Geometry: final body of the model. Coordinates: model frame, mm. Give positions to 0.01 mm unless a question says otherwise; leave off trailing zeros. Loops run counter-clockwise (first coordinate to the right, second up) from the corner with the lowest first, then second, coordinate; pieces in that order, holes last. Notation, with made-up numbers: (87, -10) -> (95, -10) arc R18 ccw to (95, -5) -> close; hole circle Ø4 at (68, 60.25). An arc over 180 degrees is marked (long way). One line per question, with ' | ' between items. Start each with the question number.
Item 1: Pin query (flat end, axial travel): P1, Ø4, axis at x = -24.5, y = 1.5, coming from the -Z side; P2, Ø3, axis at x = -38, y = 0, coming from the -Z side; P3, Ø1.5, axis at x = 7, y = 4, coming from the +Z side. Return the tip coordinate at first contact, or that it passes through.
Item 2: Material intervals for line 1 along Y through (x, z) = (-38, 20); line 2 along X through (y, z) = (1, 18.75); line 3 along X through (y, z) = (-2.5, 19.25), sorted ascending. Write a range as [from, to].
Item 3: Section A-A on z = 18. Return loops of the section in (x, y).
from build123d import *

# Parameters (mm, degrees)
SALIENTE_EXTRUIR2_DEPTH      = 5
CROQUIS6_R                   = 3
SALIENTE_EXTRUIR3_DEPTH      = 10
CROQUIS7_R                   = 1.75
CORTAR_EXTRUIR1_DEPTH        = 10
CHAFL_N1_SIZE                = 2
REDONDEO2_START              = -5.0000001
REDONDEO2_DEPTH              = 10.0000002
SALIENTE_EXTRUIR8_DEPTH      = 4.62
SALIENTE_EXTRUIR8_DEPTH_BACK = 4.62
CROQUIS17_R                  = 2.5


with BuildPart() as part:
    # Croquis5 → Saliente-Extruir2 (new, symmetric)
    with BuildSketch(Plane(origin=(0, 0, 0), x_dir=(1, 0, 0), z_dir=(0, 1, 0))):
        with BuildLine():
            Line((0, -26), (0, -30))
            add(Edge.make_bspline(
                [(0, -30), (3.306526268, -30), (16.53263134, -29.831217065), (35.997648536, -28.565345051), (52.057120801, -26.333176426), (58.766277483, -25.109762555), (60, -24.873829164)],
                knots=[4.71238898, 4.71238898, 4.71238898, 4.71238898, 4.810563751, 5.105088062, 5.301437603, 5.346535107, 5.346535107, 5.346535107, 5.346535107], degree=3))
            Line((60, -24.873829164), (60, -20.8))
            add(Edge.make_bspline(
                [(0, -26), (33.333333333, -26), (60, -20.8)],
                knots=[4.71238898, 4.71238898, 4.71238898, 5.355890089, 5.355890089, 5.355890089], degree=2, weights=[1, 0.948683298, 1]))
        make_face()
    extrude(amount=SALIENTE_EXTRUIR2_DEPTH, both=True)

    # Croquis6 → Saliente-Extruir3 (add)
    with BuildSketch(Plane.XY.offset(26)):
        with Locations((38, 0)):
            Circle(CROQUIS6_R)
    extrude(amount=-SALIENTE_EXTRUIR3_DEPTH)

    # Croquis7 → Cortar-Extruir1 (cut)
    with BuildSketch(Plane(origin=(0, 0, 16), x_dir=(-1, 0, 0), z_dir=(0, 0, -1))):
        with Locations((-38, 0)):
            Circle(CROQUIS7_R)
    extrude(amount=-CORTAR_EXTRUIR1_DEPTH, mode=Mode.SUBTRACT)

    # Chaflán1
    chafl_n1_edges = [part.edges().sort_by_distance(p)[0] for p in [
        (60, -5, 22.836914582),
        (60, 5, 22.836914582),
        (30.12007931, -5, 28.805559056),
        (30.12007931, 5, 28.805559056),
    ]]
    chamfer(chafl_n1_edges, length=CHAFL_N1_SIZE)

    # Redondeo2: read off the stored shape, not the designer's step
    # Redondeo2 outline → Redondeo2 (cut)
    with BuildSketch(Plane(origin=(0, 0, 0), x_dir=(1, 0, 0), z_dir=(0, 1, 0)).offset(REDONDEO2_START)):
        with BuildLine():
            Line((60, -24.873829164), (60, -22.378802425))
            ThreePointArc((60, -22.378802425), (59.301153244, -24.303560526), (57.530204169, -25.331577991))
            add(Edge.make_bspline(
                [(57.530204169, -25.331577991), (58.36173126, -25.182267919), (59.185100773, -25.029668046), (60, -24.873829164)],
                knots=[5.316747273, 5.316747273, 5.316747273, 5.316747273, 5.346535107, 5.346535107, 5.346535107, 5.346535107], degree=3))
        make_face()
    extrude(amount=REDONDEO2_DEPTH, mode=Mode.SUBTRACT)

    # Croquis17 → Saliente-Extruir8 (add, two sides: drawn at the far end of the back side and taken through both)
    with BuildSketch(Plane(origin=(0, 0, 0), x_dir=(0, 0, -1), z_dir=(1, 0, 0)).offset(-SALIENTE_EXTRUIR8_DEPTH_BACK)):
        with BuildLine():
            ThreePointArc((-21.96097599, 5), (-16.96097599, 0), (-21.96097599, -5))
            Line((-21.96097599, -5), (-26.96097599, -5))
            Line((-26.96097599, -5), (-26.96097599, 5))
            Line((-26.96097599, 5), (-21.96097599, 5))
        make_face()
        with Locations((-21.96097599, 0)):
            Circle(CROQUIS17_R, mode=Mode.SUBTRACT)
    extrude(amount=SALIENTE_EXTRUIR8_DEPTH + SALIENTE_EXTRUIR8_DEPTH_BACK)

    # Simetría2: part across plane


with BuildPart() as part_1:
    add(part.part)
    add(part.part.mirror(Plane(origin=(0, 0, 0), x_dir=(0, 0, 1), z_dir=(1, 0, 0))))


solid = part_1.part
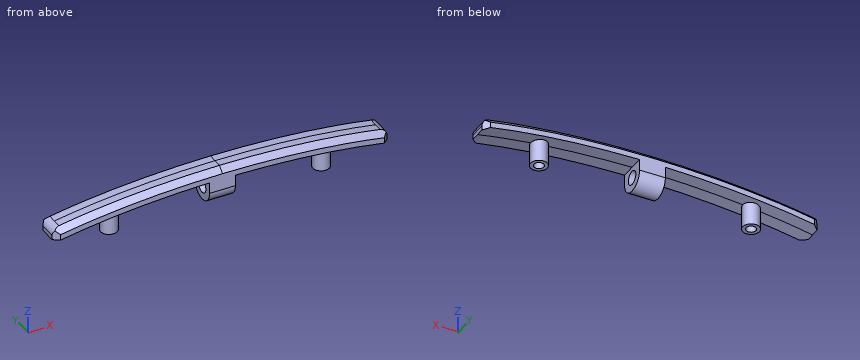
Result sheet:
1) P1: stops at z = 25.07 | P2: stops at z = 26 | P3: stops at z = 29.69
2) line 1: y = [-3, -1.75], [1.75, 3] | line 2: x = [-40.83, -39.44], [-36.56, -35.17], [-4.62, 4.62], [35.17, 36.56], [39.44, 40.83] | line 3: x = [-39.66, -36.34], [-4.62, 4.62], [36.34, 39.66]
3) outline: circle Ø6 at (-38, 0); (-4.62, -3.05) -> (4.62, -3.05) -> (4.62, 3.05) -> (-4.62, 3.05) -> close; circle Ø6 at (38, 0); hole circle Ø3.5 at (-38, 0); hole circle Ø3.5 at (38, 0)
